Input: part model. Units: mm. Frame: model coordinates. A direction names the side the tool comes from. Give positions to 0.01 mm unless a question says otherwise; leave off trailing zeros. Loops run counter-clockwise (first coordinate to the right, second up) from the corner with the lowest first, then second, coordinate; pieces in that order, holes last. Notation, with made-up numbers: (-33.75, 87.5) -> (20.25, 87.5) arc R23 ccw to (20.25, 120.5) -> close; hole circle Ø11 at (4, 46.5). An arc over 180 degrees is marked (long way). Answer as a JSON object with one key per item and string values.
```python
from build123d import *

# Parameters (mm, degrees)
F0_R       = 25.4
F1_DEPTH   = 152.4
F2_R       = 12.7
F1_FACE1_W = 304.8
F1_FACE1_H = 152.4
F3_DEPTH   = 12.7


with BuildPart() as f1:
    # F0 (on Front) → F1 (new body)
    with BuildSketch(Plane.XZ):
        with BuildLine():
            ThreePointArc((-152.4, -14.5780997561), (-165.1, -27.2780997561), (-152.4, -39.9780997561))
            Line((-152.4, -39.9780997561), (152.4, -39.9780997561))
            ThreePointArc((152.4, -39.9780997561), (165.1, -27.2780997561), (152.4, -14.5780997561))
            Line((152.4, -14.5780997561), (50.8, -14.5780997561))
            ThreePointArc((50.8, -14.5780997561), (48.4999880709, -7.2890498781), (50.8, 0))
            ThreePointArc((50.8, 0), (0, 50.8), (-50.8, 0))
            ThreePointArc((-50.8, 0), (-48.4999880709, -7.2890498781), (-50.8, -14.5780997561))
            Line((-50.8, -14.5780997561), (-152.4, -14.5780997561))
        make_face()
        Circle(F0_R, mode=Mode.SUBTRACT)
        Circle(F0_R)
    extrude(amount=F1_DEPTH)

    # F2 (on face) + F1_face1 (on face) → F3 (cut)
    with BuildSketch(Plane.XY.offset(-14.5780997561)):
        with Locations((115.9101505241, -127)):
            Circle(F2_R)
        with Locations((116.8997645463, -50.8)):
            Circle(F2_R)
        with Locations((-115.9101505241, -127)):
            Circle(F2_R)
        with Locations((-116.8997645463, -50.8)):
            Circle(F2_R)
    with BuildSketch(Plane(origin=(0, -76.2, -39.9780997561), x_dir=(1, 0, 0), z_dir=(0, 0, -1))):
        Rectangle(F1_FACE1_W, F1_FACE1_H)
    extrude(amount=-F3_DEPTH, dir=(0, 0, 1), mode=Mode.SUBTRACT)


solid = f1.part
```
Q1. Access query for faces 4 (the flat face through (-2, 0, -4)), 5 (the flat face through (102, -75, -14.578)), 6 (the cylindrical face through (127.642, -131.864, -20.839)), 7 (the flat face through (-101, -75, -14.578)). Directions: +Z, -Z, +X, -X, +Y, -Y. A direction counts if a zero-diameter tool reaches every point of the face in a straight line with its end or side. Return the directions, or none.
Evaluation:
{"face 4": "+Z, -Z, +X, -X, +Y", "face 5": "+Z, +X, +Y, -Y", "face 6": "+Z", "face 7": "+Z, -X, +Y, -Y"}
Q2. Pin query (flat end, axial travel): pin 1 (3 mm diameter, centred on x = 79, y = -31.5, fed in from +Z); pin 2 (1 mm diameter, centred on y = -79, z = 22, fed in from +X); pin 3 (6 mm diameter, centred on y = -62.5, z = 39, fed in from -X). Return the tip coordinate at first contact, or that it passes through.
Evaluation:
{"pin 1": "stops at z = -14.58", "pin 2": "stops at x = 46.03", "pin 3": "stops at x = -35.84"}
Q3. Section C-C, the plane y = -127. Return the cut outline in (x, z).
Evaluation:
{"outline": "(-152.4, -39.98) -> (152.4, -39.98) arc R12.7 ccw to (152.4, -14.58) -> (128.61, -14.58) -> (128.61, -27.28) -> (103.21, -27.28) -> (103.21, -14.58) -> (50.8, -14.58) arc R12.7 cw to (50.8, 0) arc R50.8 ccw to (-50.8, 0) arc R12.7 cw to (-50.8, -14.58) -> (-103.21, -14.58) -> (-103.21, -27.28) -> (-128.61, -27.28) -> (-128.61, -14.58) -> (-152.4, -14.58) arc R12.7 ccw to start"}
Q4. Draft query along Y for faces 1 (the flat face through (-116, -127, -27.278)), 2 (the cylindrical face through (-165.097, -75.133, -26.999)), 3 (the flat face through (-2, -152.4, -4)). Return one class per face: +Y half, -Y half, draft (parallel to the pull), parting line (faces both ways), or undercut.
Evaluation:
{"face 1": "undercut", "face 2": "draft", "face 3": "-Y half"}
Q5. Section D-D, the plane z = 37.5. Return the cut outline in (x, y), then the cut area to 3 significant figures.
Evaluation:
{"outline": "(-34.27, -152.4) -> (34.27, -152.4) -> (34.27, 0) -> (-34.27, 0) -> close", "area": "10,400 mm2"}
Q6. Section A-A, the plane y = -88. Return the cut outline in (x, z).
Evaluation:
{"outline": "(-152.4, -39.98) -> (152.4, -39.98) arc R12.7 ccw to (152.4, -14.58) -> (50.8, -14.58) arc R12.7 cw to (50.8, 0) arc R50.8 ccw to (-50.8, 0) arc R12.7 cw to (-50.8, -14.58) -> (-152.4, -14.58) arc R12.7 ccw to start"}
Q7. Ray query, line 1 along X through (y, z) = (-50, -22); line 2 along X through (y, z) = (-50, -21); line 3 along X through (y, z) = (-42, -28.5). Return the intervals inside material, ascending.
Evaluation:
{"line 1": "x = -163.95 to -129.57, -104.22 to 104.22, 129.57 to 163.95", "line 2": "x = -163.44 to -129.57, -104.22 to 104.22, 129.57 to 163.44", "line 3": "x = -165.04 to 165.04"}
Q8. Section B-B, the plane x = 56. Return the cut outline in (y, z).
Evaluation:
{"outline": "(-152.4, -39.98) -> (0, -39.98) -> (0, -14.58) -> (-152.4, -14.58) -> close"}
